from build123d import *

# Parameters (mm, degrees)
FILLET1_R     = 1.5
CHAMFER1_SIZE = 0.75
FILLET2_R     = 0.5


with BuildPart() as part:
    # Sketch2 → Revolve1 (revolve)
    with BuildSketch(Plane.XY, mode=Mode.PRIVATE) as revolve1_sk:
        Polygon((0, 0), (0, 5.5), (-2, 5.5), (-2, 3), (-12, 3), (-12, 4.5), (-13.5, 4.5), (-13.5, 3), (-16.5, 3), (-16.5, 0), align=None)
    revolve(revolve1_sk.sketch.rotate(Axis((-42.300017882, 0, 0), (1, 0, 0)), 90), axis=Axis((-42.300017882, 0, 0), (1, 0, 0)))

    # Fillet1
    fillet1_edges = [part.edges().sort_by_distance(p)[0] for p in [
        (0, 0, -5.5),
    ]]
    fillet(fillet1_edges, radius=FILLET1_R)

    # Chamfer1
    chamfer1_edges = [part.edges().sort_by_distance(p)[0] for p in [
        (-13.5, 0, -4.5),
    ]]
    chamfer(chamfer1_edges, length=CHAMFER1_SIZE)

    # Fillet2
    fillet2_edges = [part.edges().sort_by_distance(p)[0] for p in [
        (-12.75, 0, -4.5),
        (-12, 0, -4.5),
    ]]
    fillet(fillet2_edges, radius=FILLET2_R)


solid = part.part
Work out the finished part from the listing and answer in its coordinate system (mm). A direction names the side the tool comes from. Round coordinates to 2 decimals unless told otherwise and drop trailing zeros. Order: outer loops, then holes, each group sorted by start corner. A loop starts at its lowest first (then second) coordinate and runs counter-clockwise, first axis right, second up. Notation, with made-up numbers: M 88.25,-28 L 101.25,-28 A7 cw 101.25,-19 Z; hole C -24,-15 d11. An arc over 180 degrees is marked long. One line per item, written item: value.
Q1. Determine the mould class of faces 3 (the face through (-15.02, -0.9, 2.86)), 4 (the face through (-2, 2.4, 2.4)), 5 (the face through (-7.07, -0.9, 2.86)), 6 (the face through (-13.5, -3, 1)) for opening direction X: released by +X, released by -X, zero draft, split by the parting line, or undercut.
Derived:
face 3: zero draft
face 4: undercut
face 5: undercut
face 6: released by -X
Q2. Find section A-A on x = -10.5. Write down the section's boundary in (y, z).
Derived:
outline: C 0,0 d6
Q3. Straight lines are drawn through the part: line 1 (X direction, y = -3.25, z = 1.75); line 2 (X direction, y = 3.25, z = 3); line 3 (X direction, y = -4, z = 3.25). For each, find the intervals that lie inside material, in ascending order.
Derived:
line 1: -13.5 to -12, -2 to 0
line 2: -12.81 to -12.23, -2 to -0.06
line 3: -2 to -0.54
Q4. For faces 1 (the face through (-12, -3, -1)), 2 (the face through (0, 0, 0)), determine the directions among +Z, -Z, +X, -X, +Y, -Y from which every point of the face is accessible in a straight line to the end or side of a thin tool.
Derived:
face 1: none
face 2: +Z, -Z, +X, +Y, -Y
Q5. Flat-ended cylindrical pins translate along their axes: pin 1 (3 mm diameter, centred on x = -11.5, y = 0.5, fed in from -Z); pin 2 (4 mm diameter, centred on x = -2, y = 3, fed in from +Z); pin 3 (1.5 mm diameter, centred on x = -11.5, y = -3, fed in from +Z). Find the tip coordinate at first contact, or state that the pin passes through.
Derived:
pin 1: z = -4.5
pin 2: z = 5.41
pin 3: z = 3.48
